Part model, mm, in its own coordinate system. Face numbers are marked on the shaded views. A direction names the side the tool comes from. Round coordinates to 2 decimals unless told otherwise and drop trailing zeros. Order: outer loops, then holes, each group sorted by start corner. A loop starts at its lowest first (then second) coordinate and runs counter-clockwise, first axis right, second up. Notation, with made-up numbers: M -15,-9 L 7,-9 A23 cw 7,11 Z; hole C 47.5,9.5 d6. An arc over 180 degrees is marked long. Write each question's results on one line, items separated by ' | '. Start each with the question number.
1. Band-saw the part on A-A, the plane x = 0. List the corners of the cut face in (y, z), then the cut area to 4 significant figures.
2. Which spindle directions (+Z, -Z, +X, -X, +Y, -Y) get a long thin tool onto all of the face, cutting with end or side? Do the marked faces 1 and 2. Say none if no direction does.
3. Band-saw the part on D-D, the plane x = 8. List the corners of the cut face in (y, z).
4. Band-saw the part on C-C, the plane y = 0. List the corners of the cut face in (x, z), then the cut area to 3 significant figures.
5. Probe L1, parallel to Y at x = 0, z = 5.25; L2, parallel to X at y = 1, z = 6.25; L3, parallel to X at y = 0.75, z = 4.5. List the from-to ranges inside material, lowest first. Write a range as [from, to].
6. Two-plate mould, pull along Y, no slides. Class the marked faces 3, 4, 5 and 6: +Y half, -Y half, draft (parallel to the pull), parting line (faces both ways), or undercut.
7. Drop flat-ended pins along their axis: pin 1 Ø2 at (x, y) = (-8, 0) entering from -Z; pin 2 Ø1 at (y, z) = (2, 4) entering from -X; pin 3 Ø6 at (y, z) = (-10.5, 3.5) entering from +X; pin 4 Ø4 at (y, z) = (7, 8) entering from +X. Give the stop position or say it passes through.
8. Band-saw the part on B-B, the plane z = 5.5. List the corners of the cut face in (x, y), then the cut area to 3 significant figures.
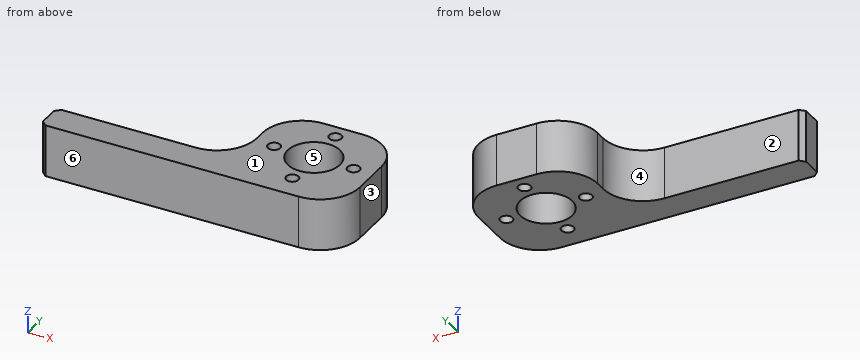
```python
from build123d import *

# Parameters (mm, degrees)
F0_R     = 1.25
F0_R_2   = 5.25
F1_DEPTH = 10.5
F2_R     = 8
F3_SIZE  = 1


with BuildPart() as f1:
    # F0 (on Top) → F1 (new body)
    with BuildSketch(Plane.XY):
        Polygon((-12, 11), (-12, -7), (-48, -7), (-48, -13), (12, -13), (12, 11), align=None)
        with Locations((0, -8)):
            Circle(F0_R, mode=Mode.SUBTRACT)
        with Locations((-8, 0)):
            Circle(F0_R, mode=Mode.SUBTRACT)
        Circle(F0_R_2, mode=Mode.SUBTRACT)
        with Locations((8, 0)):
            Circle(F0_R, mode=Mode.SUBTRACT)
        with Locations((0, 8)):
            Circle(F0_R, mode=Mode.SUBTRACT)
    extrude(amount=F1_DEPTH)

    # F2
    f2_edges = [f1.edges().sort_by_distance(p)[0] for p in [
        (12, -13, 5.25),
        (12, 11, 5.25),
        (-12, 11, 5.25),
        (-12, -7, 5.25),
    ]]
    fillet(f2_edges, radius=F2_R)

    # F3
    f3_edges = [f1.edges().sort_by_distance(p)[0] for p in [
        (-48, -13, 5.25),
        (-48, -7, 5.25),
    ]]
    chamfer(f3_edges, length=F3_SIZE)


solid = f1.part
```
Solution:
1) outline: M -13,0 L -9.25,0 L -9.25,10.5 L -13,10.5 Z; M -6.75,0 L -5.25,0 L -5.25,10.5 L -6.75,10.5 Z; M 5.25,0 L 6.75,0 L 6.75,10.5 L 5.25,10.5 Z; M 9.25,0 L 11,0 L 11,10.5 L 9.25,10.5 Z | area: 89.25 mm^2
2) face 1: +Z, +X, -X, +Y, -Y | face 2: +Z, -Z, -X, +Y
3) outline: M -11.93,0 L -1.25,0 L -1.25,10.5 L -11.93,10.5 Z; M 1.25,0 L 9.93,0 L 9.93,10.5 L 1.25,10.5 Z
4) outline: M -12.06,0 L -9.25,0 L -9.25,10.5 L -12.06,10.5 Z; M -6.75,0 L -5.25,0 L -5.25,10.5 L -6.75,10.5 Z; M 5.25,0 L 6.75,0 L 6.75,10.5 L 5.25,10.5 Z; M 9.25,0 L 12,0 L 12,10.5 L 9.25,10.5 Z | area: 89.9 mm^2
5) L1: [-13, -9.25], [-6.75, -5.25], [5.25, 6.75], [9.25, 11] | L2: [-12, -8.75], [-7.25, -5.15], [5.15, 7.25], [8.75, 12] | L3: [-12, -9], [-7, -5.2], [5.2, 7], [9, 12]
6) face 3: draft | face 4: +Y half | face 5: undercut | face 6: -Y half
7) pin 1: through | pin 2: x = -12 | pin 3: x = 11.6 | pin 4: x = 11.75
8) outline: M -48,-12 L -47,-13 L 4,-13 A8 ccw 12,-5 L 12,3 A8 ccw 4,11 L -4,11 A8 ccw -12,3 L -12,1 A8 cw -20,-7 L -47,-7 L -48,-8 Z; hole C -8,0 d2.5; hole C 0,0 d10.5; hole C 0,-8 d2.5; hole C 0,8 d2.5; hole C 8,0 d2.5 | area: 657 mm^2
